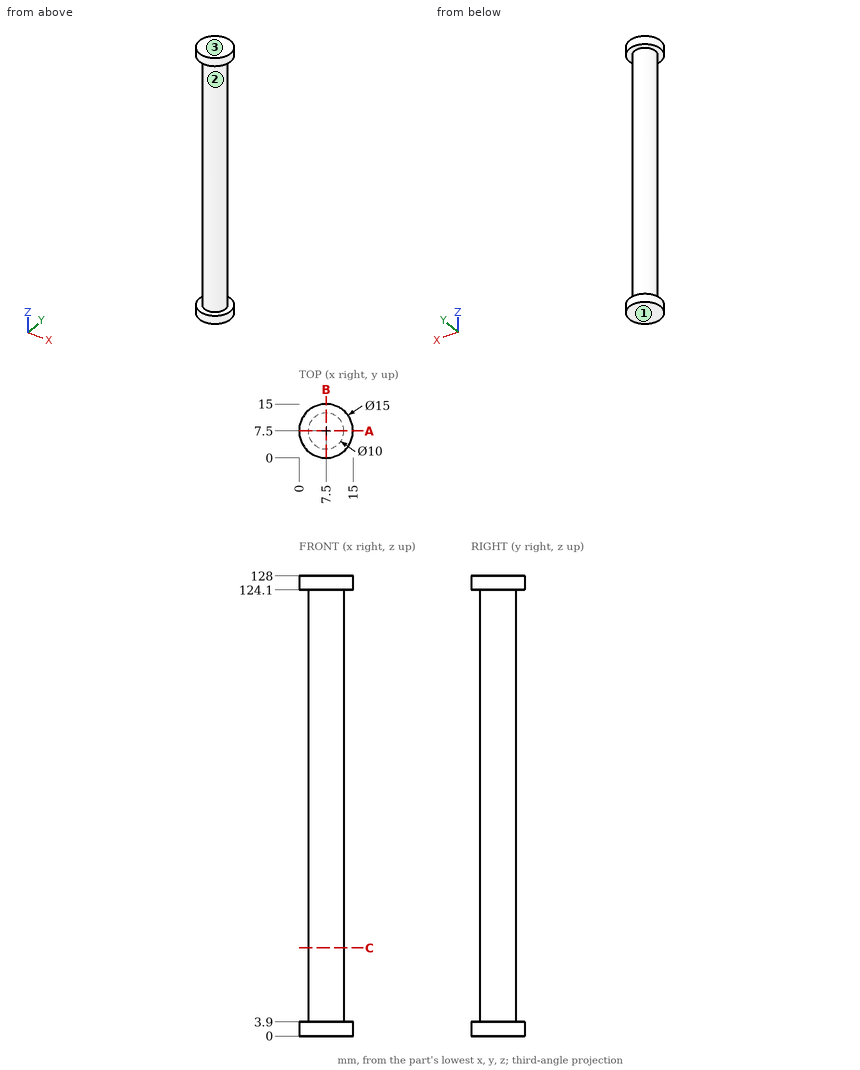
Design review of the part shown in the three views and the two pictorial views. Dimensions are in mm from the part's minimum x, y and z. Coordinates: 2 decimals unless noted, no trailing zeros. Write each loop counter-clockwise with the first axis right and the second up, starting at its lowest first coordinate (ties: lowest second). Pieces come first, ordered by that corner, then holes.
1) The part is to be moulded in two halves that separate along Z. For the marked faces 1, 2 and 3, say which applies: pulls with the +Z half, pulls with the -Z half, needs draft (parallel to the pull), parting line crosses it, or undercut.
2) Clearance check with flat-ended pins moving along their axes: pin 1 Ø2 at (x, y) = (12, 10) entering from -Z; pin 2 Ø2 at (x, z) = (7, 32.5) entering from -Y; pin 3 Ø1 at (y, z) = (13.5, 88) entering from +X; pin 4 Ø2 at (y, z) = (7, 20) entering from -X. State where each tip first meets the part, or that it passes through.
3) We need section A-A on y = 7.5. State the section outline as (x, z) points, then the cut area to 3 significant figures.
4) To check wall thickness, follow probe 1 along Z at (x, y) = (7, 2.25); probe 2 along Y at (x, z) = (7.75, 51); probe 3 along X at (y, z) = (8.25, 37). State the ranges of each line that lie inside material, in increasing order.
5) We need section C-C on z = 24.5. State the section outline as (x, y) points, then the cut area to 3 significant figures.
Answer list:
1. face 1: pulls with the -Z half
1. face 2: undercut
1. face 3: pulls with the +Z half
2. pin 1: stops at z = 0
2. pin 2: stops at y = 2.5
2. pin 3: passes through
2. pin 4: stops at x = 2.5
3. outline: (0, 0) - (15, 0) - (15, 3.9) - (12.5, 3.9) - (12.5, 124.1) - (15, 124.1) - (15, 128) - (0, 128) - (0, 124.1) - (2.5, 124.1) - (2.5, 3.9) - (0, 3.9) - close
3. area: 1,320 mm2
4. probe 1: z = 0 to 3.9, 124.1 to 128
4. probe 2: y = 2.51 to 12.49
4. probe 3: x = 2.56 to 12.44
5. outline: circle Ø10 at (7.5, 7.5)
5. area: 78.5 mm2
